Input: part model. Units: mm. Frame: model coordinates. A direction names the side the tool comes from. Round coordinates to 2 decimals unless told otherwise and drop trailing zeros. Order: outer loops, then holes, each group sorted by start corner. A loop starts at its lowest first (then second) coordinate and runs counter-clockwise, first axis right, second up. Notation, with made-up numbers: (77, 16.5) -> (98, 16.5) arc R26 cw to (98, 53.5) -> close; hole circle Ø7 at (38.5, 2). An arc over 180 degrees is marked (long way). Answer as CSV lines item,"result". Start each with the question number.
1) Line query: L1, parallel to Y at x = 22.5, z = 33; L2, parallel to Z at x = 10.5, y = -16; L3, parallel to Y at x = 8.5, z = 8.5. Output: solid intervals per line, ascending.
2) Section query D-D, the plane z = 14.5. Output: boundary loops of the cut face in (x, y).
3) Section query A-A, the plane z = 9. Output: boundary loops of the cut face in (x, y).
4) First-contact query: P1, Ø4, axis at x = -9, z = 17.5, coming from the -Y side. Flat tip, straight axial feed; report the tip coordinate or a pass-through.
5) Access query for faces 1 (the face through (-1, -22.5, 3)), 2 (the face through (-1, -17.5, 8)). Directions: +Z, -Z, +X, -X, +Y, -Y. A direction counts if a zero-diameter tool reaches every point of the face in a straight line with its end or side. Return the directions, or none.
6) Mould query, pull axis Y, two halves, no side actions, for faces 3 (the face through (0.7, 18, 44.57)), 4 (the face through (-50, 7, 4)), 5 (the face through (-1, 0, 6)). Classes: +Y half, -Y half, draft (parallel to the pull), parting line (faces both ways), or undercut.
7) Section query C-C, the plane y = -6. Output: boundary loops of the cut face in (x, z), and give its area (3 significant figures).
```python
from build123d import *

# Parameters (mm, degrees)
F0_W     = 100
F0_H     = 45
F1_DEPTH = 6
F2_W     = 100
F2_H     = 5
F3_DEPTH = 5
F4_W     = 100
F4_H     = 6
F5_DEPTH = 40
F6_R     = 4.99999
F7_R     = 5


# Not quite as in the source:
# - a fillet or chamfer is up to 0.001 mm smaller than in the source, because OpenCascade refuses the exact size


with BuildPart() as f1:
    # F0 (on Top) → F1 (new body)
    with BuildSketch(Plane.XY):
        Rectangle(F0_W, F0_H)
    extrude(amount=F1_DEPTH)

    # F2 (on face) → F3 (join)
    with BuildSketch(Plane.XY.offset(6)):
        with Locations((0, -20)):
            Rectangle(F2_W, F2_H)
    extrude(amount=F3_DEPTH)

    # F4 (on face) → F5 (join)
    with BuildSketch(Plane.XY.offset(6)):
        with Locations((0, 19.5)):
            Rectangle(F4_W, F4_H)
    extrude(amount=F5_DEPTH)

    # F6 (radius 5 in the source; OpenCascade refuses exactly that, so slightly less here)
    f6_edges = [f1.edges().sort_by_distance(p)[0] for p in [
        (0, -22.5, 11),
    ]]
    fillet(f6_edges, radius=F6_R)

    # F7
    f7_edges = [f1.edges().sort_by_distance(p)[0] for p in [
        (0, 16.5, 46),
    ]]
    fillet(f7_edges, radius=F7_R)


solid = f1.part
```
Findings:
1,L1,"y = 16.5 to 22.5"
1,L2,"z = 0 to 6"
1,L3,"y = -21.83 to -17.5, 16.5 to 22.5"
2,outline,"(-50, 16.5) -> (50, 16.5) -> (50, 22.5) -> (-50, 22.5) -> close"
3,outline,"(-50, -21.5) -> (50, -21.5) -> (50, -17.5) -> (-50, -17.5) -> close; (-50, 16.5) -> (50, 16.5) -> (50, 22.5) -> (-50, 22.5) -> close"
4,P1,"stops at y = 16.5"
5,face 1,"+Z, -Z, +X, -X, -Y"
5,face 2,"+Z, +X, -X"
6,face 3,"-Y half"
6,face 4,"draft"
6,face 5,"undercut"
7,outline,"(-50, 0) -> (50, 0) -> (50, 6) -> (-50, 6) -> close"
7,area,"600 mm^2"
